Part model, mm, in its own coordinate system. Face numbers are marked on the shaded views. A direction names the side the tool comes from. Round coordinates to 2 decimals unless told otherwise and drop trailing zeros. Loops run counter-clockwise (first coordinate to the right, second up) from the corner with the lowest first, then second, coordinate; pieces in that order, holes last.
1) Drop flat-ended pins along their axis: P1, Ø3, axis at x = -7, y = -8, coming from the -Z side; P2, Ø3, axis at x = 17.5, y = -3.5, coming from the -Z side; P3, Ø3, axis at x = 0, y = -7, coming from the +Z side; P4, Ø3, axis at x = -15.5, z = -21.5, coming from the -Y side. Give the stop position or say it passes through.
2) 3-axis set-ups, long thin cutter, end or side, ignore diameter. For the marked faces 5, 6, 7, 8 and 9: which of +Z, -Z, +X, -X, +Y, -Y reach the whole face in a straight line?
3) Mould opens along X. For the marked faces 1, 2, 3 and 4 say: +X half, -X half, draft (parallel to the pull), parting line (faces both ways), or undercut.
4) Band-saw the part on A-A, the plane z = 7.5. Write the cut outline in (x, y), then the cut area to 3 significant figures.
5) Band-saw the part on C-C, the plane z = -28. Write the cut outline in (x, y).
6) Probe line 1 (Z direction, x = -4, y = -1.75); line 2 (Z direction, x = -14.5, y = -1.5); line 3 (Z direction, x = -11, y = -6). List the from-to ranges inside material, lowest first.
7) Band-saw the part on D-D, the plane z = -37. Write the cut outline in (x, y), then the cut area to 3 significant figures.
8) Band-saw the part on B-B, the plane y = -4.5. State how many separate pieces and enclosed holes the cut face has, then the cut area to 3 significant figures.
from build123d import *

# Parameters (mm, degrees)
F1_DEPTH = 10


with BuildPart() as f1:
    # F0 (on Front) → F1 (new body)
    with BuildSketch(Plane.XZ):
        Polygon((-10.7119849175, -24.0873143706), (-6.0931825641, -24.0873143706), (-13.046591282, -12.0436571853), (-15.3559924588, -16.0436573585), align=None)
        Polygon((4.3611317565, -27.0873143706), (0, -34.6410161514), (-4.3611317565, -27.0873143706), (-8.9799341099, -27.0873143706), (0, -42.6410164977), (8.9799341099, -27.0873143706), align=None)
        Polygon((13.046591282, -12.0436571853), (6.0931825641, -24.0873143706), (10.7119849175, -24.0873143706), (15.3559924588, -16.0436573585), align=None)
        Polygon((20, 0), (14.7208913197, -9.143684453), (17.0212680072, -13.1593155), (23.4641017651, -2.0000000866), (27.1496195346, 4.00000019), (20, 4.00000019), (7.1914581155, 4.00000019), (9.4828805792, 0), align=None)
        Polygon((-3.7837813776, 4.00000019), (-6.0931825641, 0), (6.0931825641, 0), (3.7837813776, 4.00000019), align=None)
        Polygon((-17.0880432663, -13.0436573585), (-14.7786420896, -9.0436571853), (-20, 0), (-9.5572841792, 0), (-7.2478829927, 4.00000019), (-20, 4.00000019), (-26.9282035399, 4.00000019), (-23.4641017651, -2.0000000866), align=None)
        Polygon((-15.3559924588, -16.0436573585), (-13.046591282, -12.0436571853), (-14.7786420896, -9.0436571853), (-17.0880432663, -13.0436573585), align=None)
        Polygon((-8.9799341099, -27.0873143706), (-4.3611317565, -27.0873143706), (-6.0931825641, -24.0873143706), (-10.7119849175, -24.0873143706), align=None)
        Polygon((6.0931825641, -24.0873143706), (4.3611317565, -27.0873143706), (8.9799341099, -27.0873143706), (10.7119849175, -24.0873143706), align=None)
        Polygon((14.7208913197, -9.143684453), (13.046591282, -12.0436571853), (15.3559924588, -16.0436573585), (17.0212680072, -13.1593155), align=None)
        Polygon((3.7837813776, 4.00000019), (6.0931825641, 0), (9.4828805792, 0), (7.1914581155, 4.00000019), align=None)
        Polygon((-9.5572841792, 0), (-6.0931825641, 0), (-3.7837813776, 4.00000019), (-7.2478829927, 4.00000019), align=None)
        Polygon((-14.7786420896, -9.0436571853), (-13.046591282, -12.0436571853), (-6.0931825641, 0), (-9.5572841792, 0), align=None)
        Polygon((-25.1961524227, -27.0873143706), (-8.9799341099, -27.0873143706), (-10.7119849175, -24.0873143706), (-20, -24.0873143706), (-15.3559924588, -16.0436573585), (-17.0880432663, -13.0436573585), align=None)
        Polygon((-6.0931825641, -24.0873143706), (-4.3611317565, -27.0873143706), (4.3611317565, -27.0873143706), (6.0931825641, -24.0873143706), align=None)
        Polygon((10.7119849175, -24.0873143706), (8.9799341099, -27.0873143706), (25, -27.0873143706), (17.0212680072, -13.1593155), (15.3559924588, -16.0436573585), (20, -24.0873143706), align=None)
        Polygon((6.0931825641, 0), (13.046591282, -12.0436571853), (14.7208913197, -9.143684453), (9.4828805792, 0), align=None)
        Polygon((-7.2478829927, 4.00000019), (-3.7837813776, 4.00000019), (0, 10.5537017807), (3.7837813776, 4.00000019), (7.1914581155, 4.00000019), (0, 16.5537017807), align=None)
    extrude(amount=F1_DEPTH)


solid = f1.part
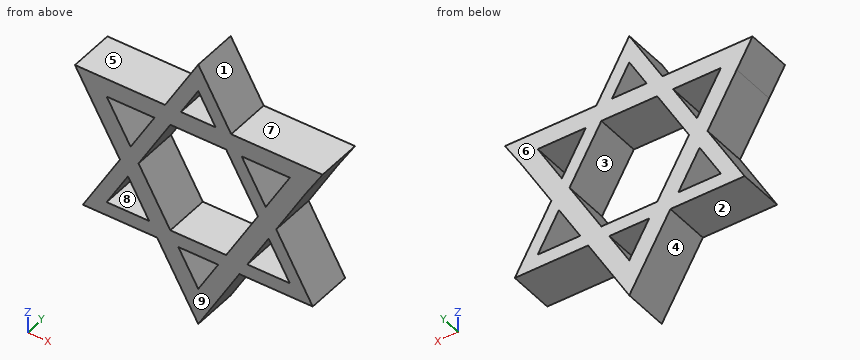
Reported:
1. P1: stops at z = -33.11
1. P2: stops at z = -27.09
1. P3: stops at z = 16.55
1. P4: passes through
2. face 5: +Z, -X, +Y, -Y
2. face 6: +Z, -Z, +X, -X, +Y
2. face 7: +Z, +X, +Y, -Y
2. face 8: +Y, -Y
2. face 9: +Z, -Z, +X, -X, -Y
3. face 1: +X half
3. face 2: draft
3. face 3: undercut
3. face 4: -X half
4. outline: (-5.23, -10) - (-1.76, -10) - (-1.76, 0) - (-5.23, 0) - close; (1.76, -10) - (5.19, -10) - (5.19, 0) - (1.76, 0) - close
4. area: 68.9 mm2
5. outline: (-8.45, -10) - (-3.83, -10) - (-3.83, 0) - (-8.45, 0) - close; (3.83, -10) - (8.45, -10) - (8.45, 0) - (3.83, 0) - close
6. line 1: z = -35.71 to -27.71, -27.09 to -24.09, 0 to 9.63
6. line 2: z = -27.09 to -24.09, -17.53 to -8.56, 0 to 4
6. line 3: z = -27.09 to -24.09, -23.59 to -15.59, -8.5 to -2.5, 0 to 4
7. outline: (-3.26, -10) - (3.26, -10) - (3.26, 0) - (-3.26, 0) - close
7. area: 65.1 mm2
8. separate pieces: 1
8. enclosed holes: 7
8. area: 884 mm2
